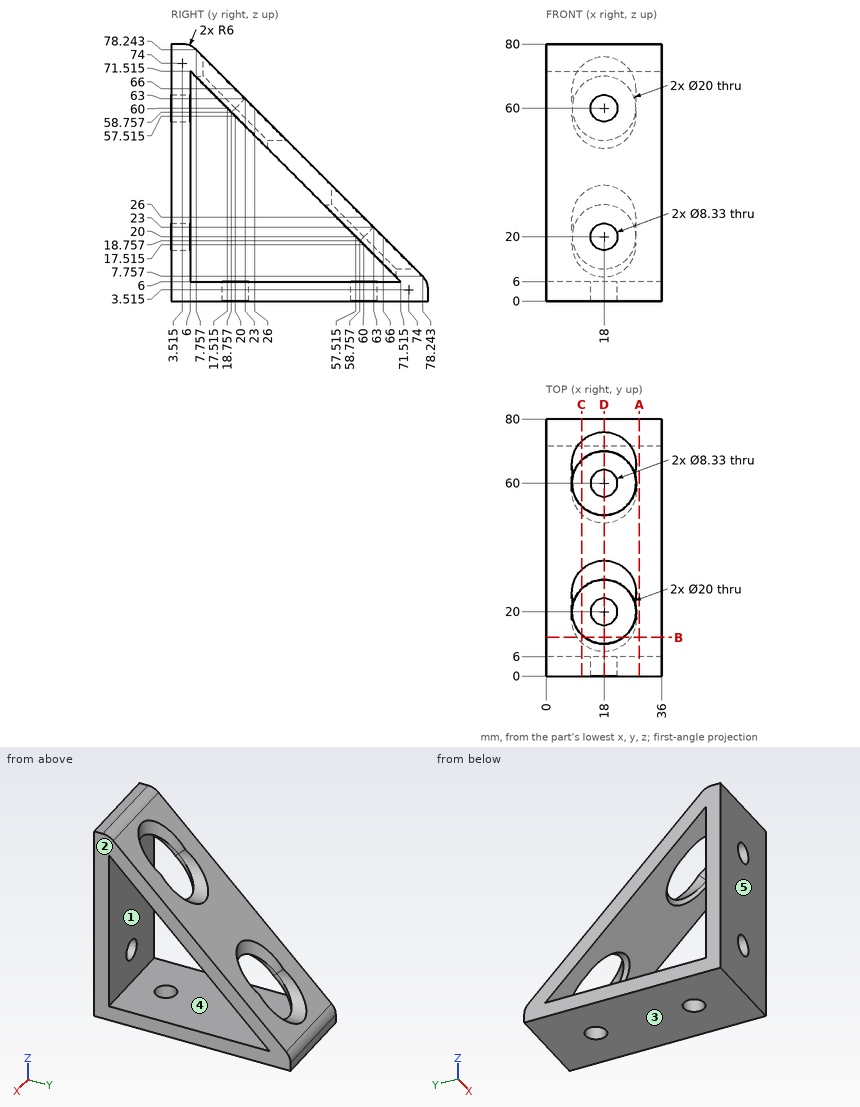
Study the drawing (mm; zero at the part's minimum x, y, z) and answer. A direction names the side the tool comes from. Give positions to 0.01 mm unless a question says otherwise; leave off trailing zeros. Loops run counter-clockwise (first coordinate to the right, second up) from the corner with the lowest first, then second, coordinate; pieces in that order, holes last. Notation, with made-up numbers: (88.25, 2.5) - (137.25, 2.5) arc R38 cw to (137.25, 41.5) - close; hole circle Ø5 at (36, 26). An arc over 180 degrees is marked (long way). One line per question, with ' | ' between items.
(1) The part is cut by section A-A (x = 29). Write down the section's boundary in (y, z) (1 decimal), then the cut area to 3 significant figures.
Recorded:
outline: (0, 0) - (80, 0) - (80, 3.5) arc R6 ccw to (78.2, 7.8) - (7.8, 78.2) arc R6 ccw to (3.5, 80) - (0, 80) - close; hole (6, 6) - (71.5, 6) - (6, 71.5) - close | area: 1,510 mm²
(2) The mould has two halves that part along Z. Classify the marked faces 3, 4 and 5: +Z half, -Z half, draft (parallel to the pull), parting line (faces both ways), or undercut.
Recorded:
face 3: -Z half | face 4: undercut | face 5: draft
(3) Each of these flat-tipped pins is pushed along its axis until it touches: pin 1 Ø1.5 at (x, y) = (30.5, 44) entering from +Z; pin 2 Ø11 at (x, y) = (18, 20) entering from +Z; pin 3 Ø1.5 at (x, z) = (29, 9) entering from +Y. Where does it stop, or does it pass through?
Recorded:
pin 1: stops at z = 42.75 | pin 2: stops at z = 6 | pin 3: stops at y = 77.75
(4) Straight lines are drawn through the part: probe 1 along Y at (x, z) = (18, 3.2) (1 decimal); probe 2 along X at (y, z) = (2.5, 60) (1 decimal). For each, find the intervals that lie inside material, in ascending order.
Recorded:
probe 1: y = 0 to 15.8, 24.2 to 55.8, 64.2 to 80 | probe 2: x = 0 to 13.8, 22.2 to 36
(5) The part is cut by section C-C (x = 11). Write down the section's boundary in (y, z) (1 decimal), then the cut area to 3 significant figures.
Recorded:
outline: (0, 0) - (80, 0) - (80, 3.5) arc R6 ccw to (78.2, 7.8) - (73.1, 12.9) - (67.1, 12.9) - (67.1, 10.4) - (71.5, 6) - (6, 6) - (6, 71.5) - (10.4, 67.1) - (12.9, 67.1) - (12.9, 73.1) - (7.8, 78.2) arc R6 ccw to (3.5, 80) - (0, 80) - close; (27.1, 50.4) - (50.4, 27.1) - (52.9, 27.1) - (52.9, 33.1) - (33.1, 52.9) - (27.1, 52.9) - close | area: 1,230 mm²
(6) The part is cut by section B-B (y = 12). Write down the section's boundary in (x, z) (1 decimal), then the cut area to 3 significant figures.
Recorded:
outline: (0, 0) - (36, 0) - (36, 6) - (0, 6) - close; (0, 65.5) - (9.7, 65.5) arc R10 cw to (12, 68) - (12, 74) - (0, 74) - close; (24, 68) arc R10 cw to (26.3, 65.5) - (36, 65.5) - (36, 74) - (24, 74) - close | area: 413 mm²
(7) The part is cut by section D-D (x = 18). Count the separate pieces of the cut face and the enclosed holes in it, then the cut area to 3 significant figures.
Recorded:
separate pieces: 6 | enclosed holes: 0 | area: 933 mm²
(8) A tool of negligible diameter and unlimited length cuts with its end or side. For the marked faces 1 and 2, from which of +Z, -Z, +X, -X, +Y, -Y can it reach the whole face along a straight path? Write none if from no direction.
Recorded:
face 1: +X, -X | face 2: +Z, -Z, +X, +Y, -Y
